from build123d import *

# Parameters (mm, degrees)
SKETCH1_W           = 170
SKETCH1_H           = 50
BOSS_EXTRUDE1_DEPTH = 2
SKETCH2_W           = 170
SKETCH2_H           = 10
BOSS_EXTRUDE2_DEPTH = 2
SKETCH3_W           = 170
SKETCH3_H           = 10
BOSS_EXTRUDE3_DEPTH = 2
SKETCH4_R           = 2.5
CUT_EXTRUDE1_DEPTH  = 2
SKETCH5_R           = 10
CUT_EXTRUDE2_DEPTH  = 0.5
SKETCH7_R           = 2
CUT_EXTRUDE4_DEPTH  = 30


with BuildPart() as part:
    # Sketch1 → Boss-Extrude1 (new body)
    with BuildSketch(Plane.XY):
        Rectangle(SKETCH1_W, SKETCH1_H)
    extrude(amount=BOSS_EXTRUDE1_DEPTH)

    # Sketch2 → Boss-Extrude2 (add)
    with BuildSketch(Plane(origin=(0, 25, 0), x_dir=(1, 0, 0), z_dir=(0, 1, 0))):
        with Locations((0, -5)):
            Rectangle(SKETCH2_W, SKETCH2_H)
    extrude(amount=-BOSS_EXTRUDE2_DEPTH)

    # Sketch3 → Boss-Extrude3 (add)
    with BuildSketch(Plane.XZ.offset(25)):
        with Locations((0, 5)):
            Rectangle(SKETCH3_W, SKETCH3_H)
    extrude(amount=-BOSS_EXTRUDE3_DEPTH)

    # Sketch4 → Cut-Extrude1 (cut)
    with BuildSketch(Plane(origin=(0, 0, 0), x_dir=(-1, 0, 0), z_dir=(0, 0, -1))):
        Circle(SKETCH4_R)
        with Locations((-50, 0)):
            Circle(SKETCH4_R)
        with Locations((50, 0)):
            Circle(SKETCH4_R)
    extrude(amount=-CUT_EXTRUDE1_DEPTH, mode=Mode.SUBTRACT)

    # Sketch5 → Cut-Extrude2 (cut)
    with BuildSketch(Plane.XY.offset(2)):
        Circle(SKETCH5_R)
    extrude(amount=-CUT_EXTRUDE2_DEPTH, mode=Mode.SUBTRACT)

    # Sketch7 → Cut-Extrude4 (cut)
    with BuildSketch(Plane(origin=(0, 0, 0), x_dir=(-1, 0, 0), z_dir=(0, 0, -1))):
        with Locations((-74.245869062, 0.225670703)):
            Circle(SKETCH7_R)
        with Locations((74.245869062, -0.225670703)):
            Circle(SKETCH7_R)
    extrude(amount=-CUT_EXTRUDE4_DEPTH, mode=Mode.SUBTRACT)


solid = part.part
The listing builds one solid part. Answer for the finished solid, in the listing's coordinates (mm). A direction names the side the tool comes from. Coordinates: 2 decimals unless noted, no trailing zeros. Order: outer loops, then holes, each group sorted by start corner. A loop starts at its lowest first (then second) coordinate and runs counter-clockwise, first axis right, second up.
Q1. For a pull along Y with two mould halves and no side action, classify faces 4 (the face through (76.244, 0.314, 0.986)), 5 (the face through (-1, 6, 0)), 6 (the face through (-1, 25, 5)), 7 (the face through (-1, -25, 5)) as pulls with the +Y half, pulls with the -Y half, needs draft (parallel to the pull), parting line crosses it, or undercut.
Q2. A cutting plane is placed at C-C, the plane y = -4.5. Write down the section's boundary in (x, z).
Q3. Consider line 1 (Y direction, x = 39.5, z = 7.25); line 2 (Y direction, x = 0, z = 1.75); line 3 (Z direction, x = 13.5, y = 5.5). Determine where each line is inside the solid, lowest interval first.
Q4. A cutting plane is placed at A-A, the plane z = 7.5. Write down the section's boundary in (x, y).
Q5. Which of the six approach directions +Z, -Z, +X, -X, +Y, -Y give full straight-line access (tool end or side, diameter ignored) to faces 1 (the face through (2, -2, 1.5)), 2 (the face through (-1, 23, 6)), 3 (the face through (85, -5.4, 1.7))?
Q6. Given P1, Ø16, axis at x = 4.5, y = -4, coming from the +Z side, flat-ended and moving along its own axis, determine where the tip first touches the part or whether it passes through.
Q7. A cutting plane is placed at D-D, the plane x = 50. Write down the section's boundary in (y, z).
Q8. A cutting plane is placed at B-B, the plane x = 0. Write down the section's boundary in (y, z), and give its area (4 significant figures).
Answers follow:
1. face 4: undercut
1. face 5: needs draft
1. face 6: pulls with the +Y half
1. face 7: pulls with the -Y half
2. outline: (-85, 0) - (85, 0) - (85, 2) - (8.93, 2) - (8.93, 1.5) - (-8.93, 1.5) - (-8.93, 2) - (-85, 2) - close
3. line 1: y = -25 to -23, 23 to 25
3. line 2: y = -25 to -10, 10 to 25
3. line 3: z = 0 to 2
4. outline: (-85, -25) - (85, -25) - (85, -23) - (-85, -23) - close; (-85, 23) - (85, 23) - (85, 25) - (-85, 25) - close
5. face 1: +Z
5. face 2: +Z, +X, -X
5. face 3: +Z, -Z, +X, +Y, -Y
6. P1: stops at z = 2
7. outline: (-25, 0) - (-2.5, 0) - (-2.5, 2) - (-23, 2) - (-23, 10) - (-25, 10) - close; (2.5, 0) - (25, 0) - (25, 10) - (23, 10) - (23, 2) - (2.5, 2) - close
8. outline: (-25, 0) - (-2.5, 0) - (-2.5, 1.5) - (-10, 1.5) - (-10, 2) - (-23, 2) - (-23, 10) - (-25, 10) - close; (2.5, 0) - (25, 0) - (25, 10) - (23, 10) - (23, 2) - (10, 2) - (10, 1.5) - (2.5, 1.5) - close
8. area: 114.5 mm2
